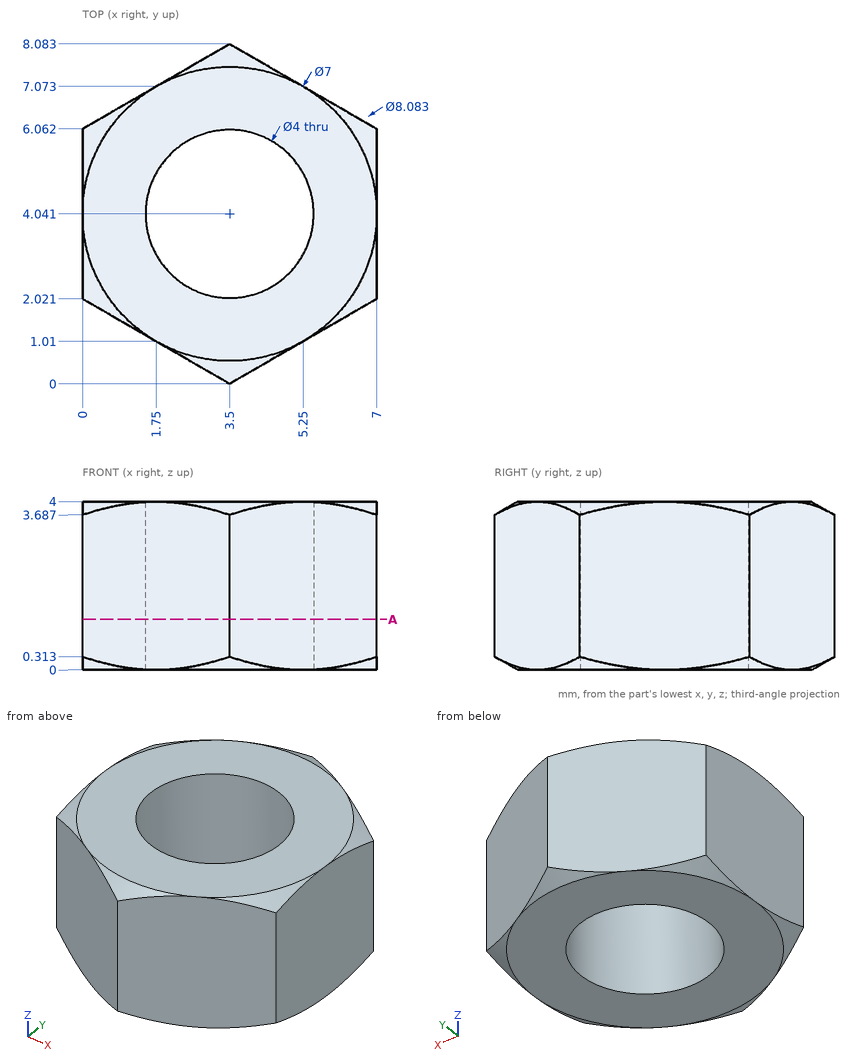
Design review of the part shown in the three views and the two pictorial views. Dimensions are in mm from the part's minimum x, y and z. Coordinates: 2 decimals unless noted, no trailing zeros. Order: outer loops, then holes, each group sorted by start corner. A loop starts at its lowest first (then second) coordinate and runs counter-clockwise, first axis right, second up. Notation, with made-up numbers: (23.25, 88.25) - (32.25, 88.25) arc R16 ccw to (32.25, 95.25) - close; hole circle Ø8 at (53, -24.5). An arc over 180 degrees is marked (long way). Answer as CSV lines item,"result". Start each with the question number.
1) To check wall thickness, follow line 1 along X through (y, z) = (4, 1.45); line 2 along Y through (x, z) = (2, 3.45) (1 decimal); line 3 along X through (y, z) = (5.25, 1.85) (1 decimal). State the ranges of each line that lie inside material, in increasing order. Write a range as [from, to].
2) Add section A-A (z = 1.2). State the section outline as (x, y) points.
3) Insertion check: P1, Ø2, axis at x = 1, z = 1, coming from the -Y side (1 decimal). The pin has a flat end and moves straight along its axis. Give the tip position at first contact, or say it passes through.
Result:
1,line 1,"[0, 1.5], [5.5, 7]"
1,line 2,"[0.9, 2.7], [5.4, 7.2]"
1,line 3,"[0, 1.9], [5.1, 7]"
2,outline,"(0, 2.02) - (3.5, 0) - (7, 2.02) - (7, 6.06) - (3.5, 8.08) - (0, 6.06) - close; hole circle Ø4 at (3.5, 4.04)"
3,P1,"y = 0.9"
